```python
from build123d import *

# Parameters (mm, degrees)
SKETCH1_R           = 4.000000000000001
SKETCH1_R_2         = 3
BOSS_EXTRUDE1_DEPTH = 2
SKETCH1_3_R         = 4.953
SKETCH1_3_R_2       = 3
BOSS_EXTRUDE2_DEPTH = 17
BOSS_EXTRUDE3_DEPTH = 10
SKETCH1_6_R         = 4.000000000000001
SKETCH1_6_R_2       = 1.500000000000002
BOSS_EXTRUDE4_DEPTH = 11.5
BOSS_EXTRUDE5_START = 2
SKETCH1_7_R         = 5.499999999999999
SKETCH1_7_R_2       = 4.000000000000001
BOSS_EXTRUDE5_DEPTH = 2.5
BOSS_EXTRUDE6_DEPTH = 2
FILLET3_R           = 0.5
FILLET4_R           = 0.5
FILLET5_R           = 0.5
FILLET6_R           = 1


with BuildPart() as part:
    # Sketch1 → Boss-Extrude1 (new body)
    with BuildSketch(Plane.XY):
        with BuildLine():
            ThreePointArc((-6.556187499999929, -11.355649853948018), (6.556187500000035, -11.355649853947956), (13.112374999999998, 2.22e-15))
            Line((13.112374999999998, 0), (13.112374999999998, 28))
            Line((13.112374999999998, 28), (4.290790826966845, 39.00080137165997))
            ThreePointArc((4.2907908269668456, 39.00080137165997), (-1.6768483404792127, 40.79814658472174), (-5.491294112785424, 35.869336332958376))
            Line((-5.491294112785426, 35.869336332958376), (-7.488128335616488, 0.42182227221597307))
            ThreePointArc((-7.488128335616491, 0.42182227221597324), (-6.5981170528310535, -3.5657890230831226), (-3.74999999999996, -6.495190528383313))
            Line((-3.74999999999996, -6.495190528383313), (-6.556187499999929, -11.355649853948018))
        make_face()
        with Locations((0, 35.559999999999995)):
            Circle(SKETCH1_R, mode=Mode.SUBTRACT)
        Circle(SKETCH1_R_2, mode=Mode.SUBTRACT)
    extrude(amount=BOSS_EXTRUDE1_DEPTH)

    # Sketch1<3> → Boss-Extrude2 (add)
    with BuildSketch(Plane.XY):
        Circle(SKETCH1_3_R)
        Circle(SKETCH1_3_R_2, mode=Mode.SUBTRACT)
    extrude(amount=BOSS_EXTRUDE2_DEPTH)

    # Sketch1<5> → Boss-Extrude3 (add)
    with BuildSketch(Plane.XY):
        with BuildLine():
            Line((10.112375, 28), (10.112375, 0))
            ThreePointArc((10.112375, -8.9e-16), (5.056187500000027, -8.757573642594647), (-5.056187499999945, -8.757573642594695))
            Line((-5.056187499999945, -8.757573642594695), (-6.556187499999929, -11.355649853948018))
            ThreePointArc((-6.556187499999929, -11.355649853948018), (6.556187500000035, -11.355649853947956), (13.112374999999998, 2.22e-15))
            Line((13.112374999999998, 0), (13.112374999999998, 28))
            Line((13.112374999999998, 28), (10.112375, 28))
        make_face()
    extrude(amount=BOSS_EXTRUDE3_DEPTH)

    # Sketch1<6> → Boss-Extrude4 (add)
    with BuildSketch(Plane.XY):
        with Locations((0, 35.559999999999995)):
            Circle(SKETCH1_6_R)
        with Locations((0, 35.559999999999995)):
            Circle(SKETCH1_6_R_2, mode=Mode.SUBTRACT)
    extrude(amount=BOSS_EXTRUDE4_DEPTH)

    # Sketch1<7> → Boss-Extrude5 (add)
    with BuildSketch(Plane.XY.offset(BOSS_EXTRUDE5_START)):
        with Locations(Location((0, 35.559999999999995, 0), (0, 0, 176.775813858))):
            Circle(SKETCH1_7_R)
        with Locations((0, 35.559999999999995)):
            Circle(SKETCH1_7_R_2, mode=Mode.SUBTRACT)
    extrude(amount=BOSS_EXTRUDE5_DEPTH)

    # Sketch3 → Boss-Extrude6 (add)
    with BuildSketch(Plane.XY.offset(2)):
        Polygon((-1, 30.151673086804013), (1, 30.151673086804013), (0.9999999999999977, 4.851000824572183), (-0.9999999999999977, 4.851000824572183), align=None)
    extrude(amount=BOSS_EXTRUDE6_DEPTH)

    # Fillet3
    fillet3_edges = [part.edges().sort_by_distance(p)[0] for p in [
        (10.112375, 28, 6),
        (13.112374999999998, 28, 6),
    ]]
    fillet(fillet3_edges, radius=FILLET3_R)

    # Fillet4
    fillet4_edges = [part.edges().sort_by_distance(p)[0] for p in [
        (13.112374999999998, 28, 1),
    ]]
    fillet(fillet4_edges, radius=FILLET4_R)

    # Fillet5
    fillet5_edges = [part.edges().sort_by_distance(p)[0] for p in [
        (-6.556187499999929, -11.355649853948018, 5),
        (-3.7499999999999605, -6.495190528383313, 1),
        (-5.056187499999946, -8.757573642594695, 6),
    ]]
    fillet(fillet5_edges, radius=FILLET5_R)

    # Fillet6
    fillet6_edges = [part.edges().sort_by_distance(p)[0] for p in [
        (-1, 30.151673086804013, 3),
        (-0.9999999999999977, 4.851000824572183, 3),
        (0.9999999999999977, 4.851000824572183, 3),
        (1, 30.151673086804013, 3),
    ]]
    fillet(fillet6_edges, radius=FILLET6_R)


solid = part.part
```
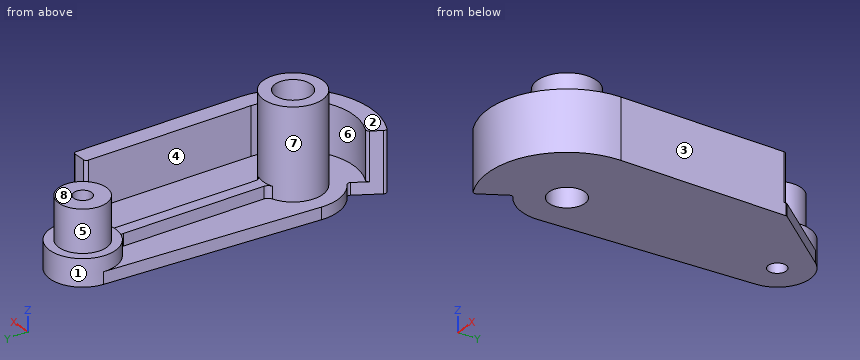
For this review, take the finished solid that the model builds, in its own axes (mm). Face numbers are marked on the shaded views. A direction names the side the tool comes from. Coordinates: 2 decimals unless noted, no trailing zeros. Write each loop counter-clockwise with the first axis right and the second up, starting at its lowest first coordinate (ties: lowest second). Pieces come first, ordered by that corner, then holes. Notation, with made-up numbers: (36, -19.5) -> (90, -19.5) arc R17 cw to (90, 9.5) -> close; hole circle Ø11 at (-33, -26.5). An arc over 180 degrees is marked (long way). Put each result on its own line as item: value.
Q1. Wall thickness on L1, parallel to Y at x = 0, z = 10.25; L2, parallel to Y at x = 0, z = 8; L3, parallel to Y at x = 0, z = 12.5: over which ranges is each line inside the solid? List them lowest first.
From the geometry:
L1: y = -4.95 to -3, 3 to 4.95, 31.56 to 34.06, 37.06 to 39.56
L2: y = -13.11 to -10.11, -4.95 to -3, 3 to 4.95, 31.56 to 34.06, 37.06 to 39.56
L3: y = -4.95 to -3, 3 to 4.95
Q2. Take a section at C-C, the plane x = -2.25. State the section outline as (y, z) points, then the cut area to 3 significant figures.
From the geometry:
outline: (-12.92, 0) -> (-1.98, 0) -> (-1.98, 17) -> (-4.41, 17) -> (-4.41, 2) -> (-9.86, 2) -> (-9.86, 10) -> (-12.92, 10) -> close; (1.98, 0) -> (40.58, 0) -> (40.58, 4.5) -> (38.87, 4.5) -> (38.87, 11.5) -> (32.25, 11.5) -> (32.25, 4.5) -> (30.54, 4.5) -> (30.54, 2) -> (4.41, 2) -> (4.41, 17) -> (1.98, 17) -> close
area: 268 mm2
Q3. Take a section at B-B, the plane x = 0. State the section outline as (y, z) points, then the cut area to 3 significant figures.
From the geometry:
outline: (-13.11, 0) -> (-3, 0) -> (-3, 17) -> (-4.95, 17) -> (-4.95, 2) -> (-10.11, 2) -> (-10.11, 10) -> (-13.11, 10) -> close; (3, 0) -> (34.06, 0) -> (34.06, 11.5) -> (31.56, 11.5) -> (31.56, 4.5) -> (30.06, 4.5) -> (30.06, 4) -> (4.95, 4) -> (4.95, 17) -> (3, 17) -> close; (37.06, 0) -> (41.06, 0) -> (41.06, 4.5) -> (39.56, 4.5) -> (39.56, 11.5) -> (37.06, 11.5) -> close
area: 278 mm2
Q4. Take a section at A-A, the plane z = 6. State the section outline as (x, y) points.
From the geometry:
outline: (-6.3, -10.91) arc R0.5 ccw to (-6.1, -11.61) arc R13.11 ccw to (13.11, 0) -> (13.11, 27.5) arc R0.5 ccw to (12.61, 28) -> (10.61, 28) arc R0.5 ccw to (10.11, 27.5) -> (10.11, 0) arc R10.11 cw to (-4.64, -8.99) arc R0.5 ccw to (-5.3, -9.18) -> close; circle Ø9.91 at (0, 0); circle Ø8 at (0, 35.56); hole circle Ø6 at (0, 0); hole circle Ø3 at (0, 35.56)
Q5. Tool access review of the marked faces 1, 2, 3 and 4: name each direction out of +Z, -Z, +X, -X, +Y, -Y from which nothing blocks a thin tool from reaching the whole face with its end or side.
From the geometry:
face 1: +Z
face 2: +Z, +X, -Y
face 3: +Z, -Z, +X, +Y, -Y
face 4: +Z, +Y
Q6. Clearance check with flat-ended pins moving along their axes: pin 1 Ø6.5 at (y, z) = (16, 6.5) entering from -X; pin 2 Ø6.5 at (x, y) = (-2, 36) entering from +Z; pin 3 Ø8 at (y, z) = (-6, 8.5) entering from -X. State where each tip first meets the part, or that it passes through.
From the geometry:
pin 1: stops at x = -1
pin 2: stops at z = 11.5
pin 3: stops at x = -5.77
Q7. The part is to be moulded in two halves that separate along X. For the marked faces 5, 6, 7 and 8, say which applies: +X half, -X half, draft (parallel to the pull), parting line (faces both ways), or undercut.
From the geometry:
face 5: parting line
face 6: undercut
face 7: undercut
face 8: draft
Q8. Take a section at D-D, the plane y = 25.5. State the section outline as (x, z) points, then the cut area to 3 significant figures.
From the geometry:
outline: (-6.08, 0) -> (13.11, 0) -> (13.11, 10) -> (10.11, 10) -> (10.11, 2) -> (1, 2) -> (1, 4) -> (-1, 4) -> (-1, 2) -> (-6.08, 2) -> close
area: 66.4 mm2
